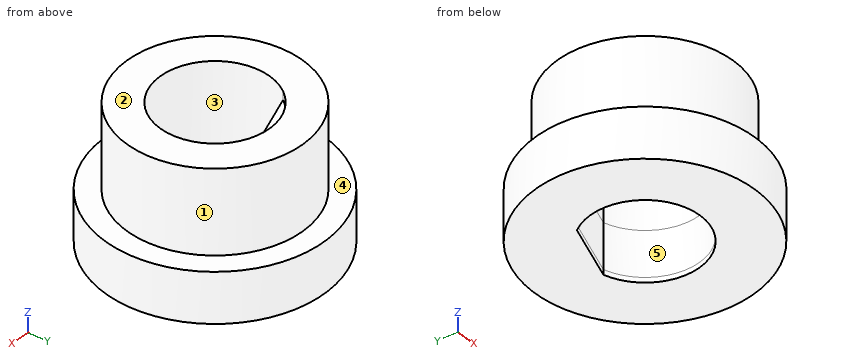
Autodesk Inventor part; units mm, degrees
ref_plane "YZ Plane" through (0, 0, 0) normal (1, 0, 0) x (0, 1, 0)
ref_plane "XZ Plane" through (0, 0, 0) normal (0, 1, 0) x (-1, 0, 0)
ref_plane "XY Plane" through (0, 0, 0) normal (0, 0, 1) x (1, 0, 0)
ref_plane "Work Plane1" through (-3.2804, 8.4734, 7) normal (0, 0, -1) x (0.3299562, -0.9439962, 0)
sketch "Sketch5" plane through (-3.2804, 8.4734, 7) normal (0, 0, -1) x (0.3299562, -0.9439962, 0)
  circle A0 centre (9.0812, -0.3009) radius 5.6
  circle A1 centre (9.0812, -0.3009) radius 6.6
  point P0 (9.0812, -0.3009)
  dimension "d13" = 1
extrude "Extrusion4" add sketch "Sketch5" along normal blind 3
sketch "Sketch6" plane through (0, 0, 7) normal (0, 0, 1) x (1, 0, 0)
  circle A0 centre (0, 0) radius 6.6
  circle A1 centre (0, 0) radius 5.6
  point P0 (0, 0)
extrude "Extrusion5" cut sketch "Sketch6" against normal blind 0.3
sketch "Sketch11" plane through (-3.2804, 8.4734, 7) normal (0, 0, -1) x (0.3299562, -0.9439962, 0)
  circle A0 centre (9.0812, -0.3009) radius 6.6
  circle A1 centre (9.0812, -0.3009) radius 3.3
  line L0 (6.3698, -2.1819) -> (6.3698, 1.5801)
  dimension "d26" = 13.2
  dimension "d27" = 6.6
  dimension "d28" = 3.762
extrude "Extrusion10" add sketch "Sketch11" along normal blind 2.7 contours A0 | L0 A1 picked at (6.2456, 0.0906)
sketch "Sketch13" plane through (-3.2804, 8.4734, 7) normal (0, 0, -1) x (0.3299562, -0.9439962, 0)
  circle A0 centre (9.0812, -0.3009) radius 5.3
  arc A1 (6.3703, -2.1826) -> (6.3703, 1.5809) centre (9.0812, -0.3009) ccw
  line L0 (6.3703, 1.5809) -> (6.3703, -2.1826)
  dimension "d33" = 10.6
extrude "Extrusion12" add sketch "Sketch13" against normal blind 5
sketch "Sketch14" plane through (0, 0, 4) normal (0, 0, -1) x (-1, 0, 0)
  line L0 (-0.881, 3.1802) -> (2.6703, 1.9389)
  arc A0 (-0.881, 3.1802) -> (2.6703, 1.9389) centre (0, 0) ccw
  circle A1 centre (0, 0) radius 5.6
  point P0 (0, 0)
extrude "Extrusion13" add sketch "Sketch14" against normal up to surface (0.3 mm away)
sketch "Sketch15" plane through (0, 0, 12) normal (0, 0, 1) x (1, 0, 0)
  arc A0 (-2.6708, 1.9382) -> (0.8818, 3.18) centre (0, 0) ccw
  circle A1 centre (0, 0) radius 3.3
  point P0 (0, 0)
extrude "Extrusion14" cut sketch "Sketch15" against normal blind 0.5
properties part number "BlankLargeGearMotorInput"
CAD build for the part. Positions are in the model's coordinates, mm. Face numbers are marked on the shaded views. A direction names the side the tool comes from. Give positions to 0.01 mm unless a question says otherwise; leave off trailing zeros. Write each loop counter-clockwise with the first axis right and the second up, starting at its lowest first coordinate (ties: lowest second). Pieces come first, ordered by that corner, then holes. Notation, with made-up numbers: M 72.5,55 L 117.5,55 A16 cw 117.5,61 Z; hole C -1,8.25 d4. An arc over 180 degrees is marked long. Put each result on its own line as item: value. Start each with the question number.
(1) Band-saw the part on C-C, the plane y = -3.5. Write the cut outline in (x, z), and give its area (3 significant figures).
(2) Probe L1, parallel to X at y = 0, z = 4.1; L2, parallel to Z at x = 4.5, y = 4; L3, parallel to Y at x = -2.5, z = 11.75. List the from-to ranges inside material, lowest first.
(3) Mould opens along X. For the marked faces 1, 2 and 3 say: +X half, -X half, draft (parallel to the pull), parting line (faces both ways), or undercut.
(4) Band-saw the part on D-D, the plane x = 4.75. Write the cut outline in (y, z), and give its area (3 significant figures).
(5) Band-saw the part on B-B, the plane z = 5.5. Write the cut outline in (x, y), and give its area (3 significant figures).
(6) Flat gauge pin, fed straight in: pin 1 Ø1.5 at (y, z) = (4.5, 7.5) entering from +X. Where does the tip first touch, or does it go through?
(7) Which spindle directions (+Z, -Z, +X, -X, +Y, -Y) get a long thin tool onto all of the face, cutting with end or side? Do the marked faces 4 and 5. Say none if no direction does.
Response values:
1. outline: M -5.6,4 L 5.6,4 L 5.6,7 L 3.98,7 L 3.98,12 L -3.98,12 L -3.98,7 L -5.6,7 Z
1. area: 73.4 mm2
2. L1: x = -6.6 to -3.3, 3.3 to 6.6
2. L2: z = 4 to 7
2. L3: y = -4.67 to -2.15, 2.15 to 4.67
3. face 1: parting line
3. face 2: draft
3. face 3: undercut
4. outline: M -4.58,4 L 4.58,4 L 4.58,7 L 2.35,7 L 2.35,12 L -2.35,12 L -2.35,7 L -4.58,7 Z
4. area: 51.0 mm2
5. outline: C 0,0 d13.2; hole M -2.67,1.94 A3.3 ccw long 0.88,3.18 Z
5. area: 104 mm2
6. pin 1: stops at x = 5.29
7. face 4: +Z
7. face 5: +Z, -Z
